Here's how the part is built. I have some questions about the finished solid (model axes, mm). A direction names the side the tool comes from. Coordinates: 2 decimals unless noted, no trailing zeros. Loops run counter-clockwise (first coordinate to the right, second up) from the corner with the lowest first, then second, coordinate; pieces in that order, holes last. Notation, with made-up numbers: (18.25, 48) -> (41.25, 48) arc R14 cw to (41.25, 75) -> close; hole circle Ø2 at (-10.75, 1.25). An arc over 180 degrees is marked (long way). Answer as a JSON object with one key per item and string values. Group by question number.
1) I need wall thicknesses on probe 1 along Y at (x, z) = (8.35, 0); probe 2 along Y at (x, z) = (1.75, 0). Which ranges of each line are inside material? Lowest first, please. Write a range as [from, to].
2) I want a section at B-B (y = 0). Write out the boundary of the cut face in (x, z).
3) If we mould it in two halves opening along Y, with no side actions, what happens to faces 4 (the flat face through (13, 0, -3.377)), 5 (the cylindrical face through (12.04, 0.07, 1.5)), 6 (the flat face through (12.535, -2.939, -1.665))? For each: +Y half, -Y half, draft (parallel to the pull), parting line (faces both ways), or undercut.
4) I want a section at C-C (z = -3.75). Write out the boundary of the cut face in (x, y), then the cut area to 3 significant figures.
5) I want a section at A-A (x = 12.5). Write out the boundary of the cut face in (y, z).
6) I'm going to push flat-ended pins straight in: pin 1 (3 mm diameter, centred on x = 13.5, y = 0, fed in from +Z); pin 2 (2 mm diameter, centred on x = 7.5, y = 3.5, fed in from +Z); pin 3 (2.5 mm diameter, centred on y = 0, z = 0, fed in from -X). Where does each tip first touch, or does it pass through?
7) Which directions (+Z, -Z, +X, -X, +Y, -Y) give clear straight access to the entire face, cutting with the end or side of a thin tool? Please do faces 1 (the flat face through (12.535, 2.911, -1.712)), 2 (the cylindrical face through (3.13, 1.34, 0.85)), 3 (the flat face through (13, 0, 3.377)).
8) I want a section at D-D (x = 7.25). Write out the boundary of the cut face in (y, z), then the cut area to 3 significant figures.
```python
from build123d import *

# Parameters (mm, degrees)
SKETCH2_OUTSIDE_W               = 22.196
SKETCH2_OUTSIDE_H               = 22.196
CUT_EXTRUDE1_DEPTH              = 5
M3X0_5_TAPPED_HOLE4_D           = 2.5
M3X0_5_TAPPED_HOLE4_DEPTH       = 8.5
M3X0_5_TAPPED_HOLE4_CBORE_D     = 3
M3X0_5_TAPPED_HOLE4_CBORE_DEPTH = 6
M3X0_5_TAPPED_HOLE4_TIP         = 0.751075774
SKETCH7_R                       = 1.58496
CUT_EXTRUDE2_DEPTH              = 6.35


with BuildPart() as part:
    # Sketch1 → Revolve1 (revolve)
    with BuildSketch(Plane(origin=(0, 0, 0), x_dir=(1, 0, 0), z_dir=(0, 1, 0))):
        Polygon((1.5, 4), (15, 4), (15, 0), (0, 0), (0, 7.5), (1.5, 7.5), align=None)
    revolve(axis=Axis((15, 0, 0), (-1, 0, 0)))

    # Sketch2 outside → Cut-Extrude1 (cut)
    with BuildSketch(Plane(origin=(15, 0, 0), x_dir=(0, 0, -1), z_dir=(1, 0, 0))):
        Rectangle(SKETCH2_OUTSIDE_W, SKETCH2_OUTSIDE_H)
        Polygon((0, 3.9), (-3.377499075, 1.95), (-3.377499075, -1.95), (0, -3.9), (3.377499075, -1.95), (3.377499075, 1.95), align=None, mode=Mode.SUBTRACT)
    extrude(amount=-CUT_EXTRUDE1_DEPTH, mode=Mode.SUBTRACT)

    # M3x0.5 Tapped Hole4
    with Locations(Plane(origin=(15, 0, 0), x_dir=(0, 0, -1), z_dir=(1, 0, 0))):
        with Locations((0, 0)):
            CounterBoreHole(M3X0_5_TAPPED_HOLE4_D / 2, M3X0_5_TAPPED_HOLE4_CBORE_D / 2, M3X0_5_TAPPED_HOLE4_CBORE_DEPTH, depth=M3X0_5_TAPPED_HOLE4_DEPTH)
            with Locations((0, 0, -(M3X0_5_TAPPED_HOLE4_DEPTH + M3X0_5_TAPPED_HOLE4_TIP / 2))):  # 118° drill point
                Cone(0, M3X0_5_TAPPED_HOLE4_D / 2, M3X0_5_TAPPED_HOLE4_TIP, mode=Mode.SUBTRACT)

    # Sketch7 → Cut-Extrude2 (cut)
    with BuildSketch(Plane.ZY):
        Circle(SKETCH7_R)
    extrude(amount=-CUT_EXTRUDE2_DEPTH, mode=Mode.SUBTRACT)


solid = part.part
```
Determined:
{
 "1": {"probe 1": "[-4, -1.25], [1.25, 4]", "probe 2": "[-4, -1.58], [1.58, 4]"},
 "2": {"outline": "(0, -7.5) -> (1.5, -7.5) -> (1.5, -4) -> (10, -4) -> (10, -3.38) -> (15, -3.38) -> (15, -1.5) -> (9, -1.5) -> (9, -1.25) -> (6.5, -1.25) -> (6.35, -1) -> (6.35, -1.58) -> (0, -1.58) -> close; (0, 1.58) -> (6.35, 1.58) -> (6.35, 1) -> (6.5, 1.25) -> (9, 1.25) -> (9, 1.5) -> (15, 1.5) -> (15, 3.38) -> (10, 3.38) -> (10, 4) -> (1.5, 4) -> (1.5, 7.5) -> (0, 7.5) -> close"},
 "3": {"face 4": "draft", "face 5": "undercut", "face 6": "-Y half"},
 "4": {"outline": "(0, -6.5) -> (1.5, -6.5) -> (1.5, -1.39) -> (10, -1.39) -> (10, 1.39) -> (1.5, 1.39) -> (1.5, 6.5) -> (0, 6.5) -> close", "area": "43.1 mm^2"},
 "5": {"outline": "(-3.9, 0) -> (-1.95, -3.38) -> (1.95, -3.38) -> (3.9, 0) -> (1.95, 3.38) -> (-1.95, 3.38) -> close; hole circle Ø3 at (0, 0)"},
 "6": {"pin 1": "z = 3.38", "pin 2": "z = 3.12", "pin 3": "x = 6.35"},
 "7": {"face 1": "-Z, +X, +Y", "face 2": "-X", "face 3": "+Z, +X, +Y, -Y"},
 "8": {"outline": "circle Ø8 at (0, 0); hole circle Ø2.5 at (0, 0)", "area": "45.4 mm^2"}
}
